Input: dimensioned drawing with shaded views. Units: mm. Origin: part minimum x, y, z. A direction names the side the tool comes from. Give positions to 0.01 mm unless a question says otherwise; leave off trailing zeros. Order: outer loops, then holes, each group sorted by start corner. A loop starts at its lowest first (then second) coordinate and runs counter-clockwise, first axis right, second up. Notation, with made-up numbers: (71.5, 37.25) - (112.5, 37.25) arc R25 ccw to (112.5, 71.25) - close; hole circle Ø11 at (-5, -21). An arc over 180 degrees is marked (long way). Use a Markdown table: item, result.
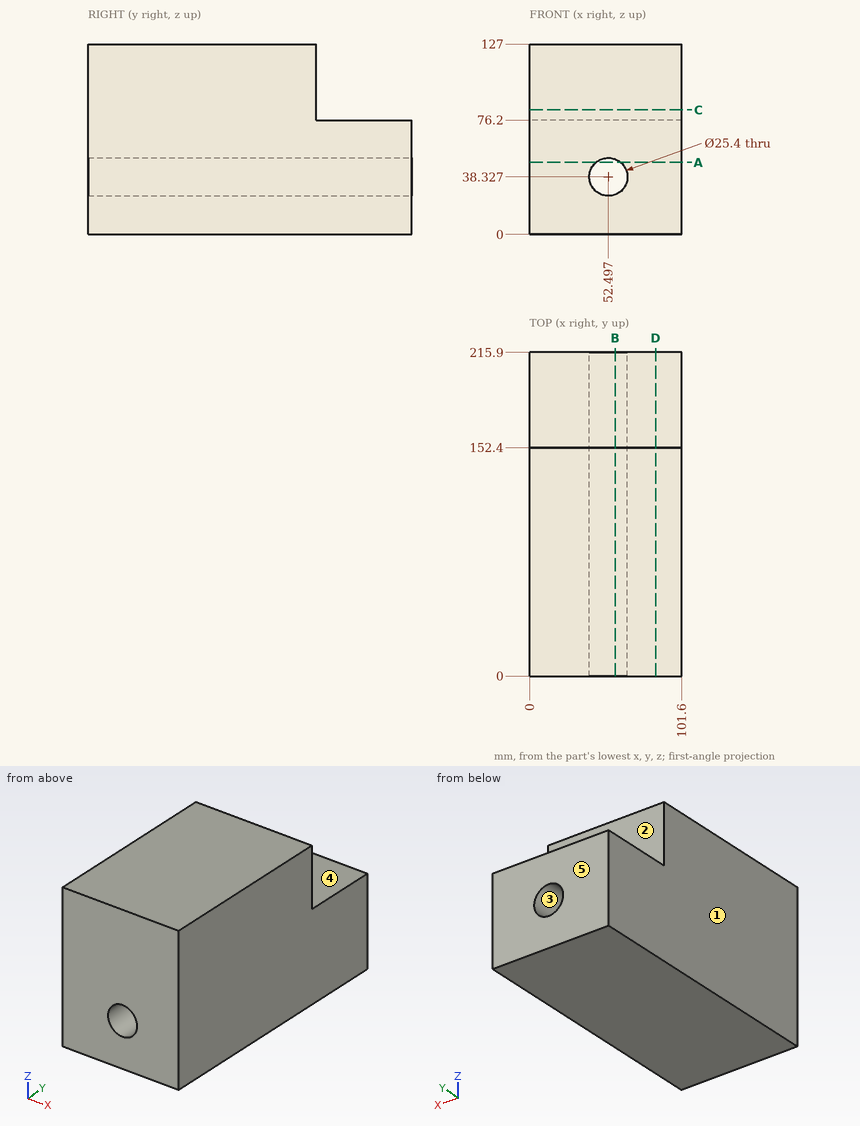
1. Section query D-D (x = 84). Return loops of the section in (y, z).
Response:
| item | result |
|---|---|
| outline | (0, 0) - (215.9, 0) - (215.9, 76.2) - (152.4, 76.2) - (152.4, 127) - (0, 127) - close |
2. Material intervals for line 1 along Y through (x, z) = (56.5, 120); line 2 along Z through (x, y) = (94, 194); line 3 along Z through (x, y) = (41, 108) (1 decimal), sorted ascending.
Response:
| item | result |
|---|---|
| line 1 | y = 0 to 152.4 |
| line 2 | z = 0 to 76.2 |
| line 3 | z = 0 to 32.9, 43.7 to 127 |
3. Section query B-B (x = 57). Return loops of the section in (y, z).
Response:
| item | result |
|---|---|
| outline | (0, 0) - (215.9, 0) - (215.9, 26.45) - (0, 26.45) - close; (0, 50.2) - (215.9, 50.2) - (215.9, 76.2) - (152.4, 76.2) - (152.4, 127) - (0, 127) - close |
4. Mould query, pull axis X, two halves, no side actions, for the marked faces 1, 2 and 3. Classes: pulls with the +X half, pulls with the -X half, needs draft (parallel to the pull), parting line crosses it, or undercut.
Response:
| item | result |
|---|---|
| face 1 | pulls with the -X half |
| face 2 | needs draft |
| face 3 | undercut |
5. Set-up query: the marked faces 4 and 5. Return all of +Z, -Z, +X, -X, +Y, -Y with unobstructed straight access to the full face (end or side cutting, diameter ignored); none if empty.
Response:
| item | result |
|---|---|
| face 4 | +Z, +X, -X, +Y |
| face 5 | +Z, -Z, +X, -X, +Y |
6. Section query A-A (z = 48). Return loops of the section in (x, y), then the cut area to 3 significant figures.
Response:
| item | result |
|---|---|
| outline | (0, 0) - (44.27, 0) - (44.27, 215.9) - (0, 215.9) - close; (60.73, 0) - (101.6, 0) - (101.6, 215.9) - (60.73, 215.9) - close |
| area | 18,400 mm^2 |
7. Pin query (flat end, axial travel): pin 1 (5 mm diameter, centred on x = 58, y = 192.5, fed in from +Z). Return the tip coordinate at first contact, or that it passes through.
Response:
| item | result |
|---|---|
| pin 1 | stops at z = 76.2 |
8. Section query C-C (z = 83). Return loops of the section in (x, y), then the cut area to 3 significant figures.
Response:
| item | result |
|---|---|
| outline | (0, 0) - (101.6, 0) - (101.6, 152.4) - (0, 152.4) - close |
| area | 15,500 mm^2 |
